Could you check a few things on this drawing? It's one solid part, dimensions in mm from its lowest x, y, z. A direction names the side the tool comes from. Round coordinates to 2 decimals unless told otherwise and drop trailing zeros. Write each loop counter-clockwise with the first axis right and the second up, starting at its lowest first coordinate (ties: lowest second). Pieces come first, ordered by that corner, then holes. Notation, with made-up numbers: (54.25, 20) -> (84.25, 20) arc R21 ccw to (84.25, 31) -> close; hole circle Ø7 at (70, -14.75). An arc over 180 degrees is marked (long way). Answer in a Markdown table with one row per item. Add a question column.
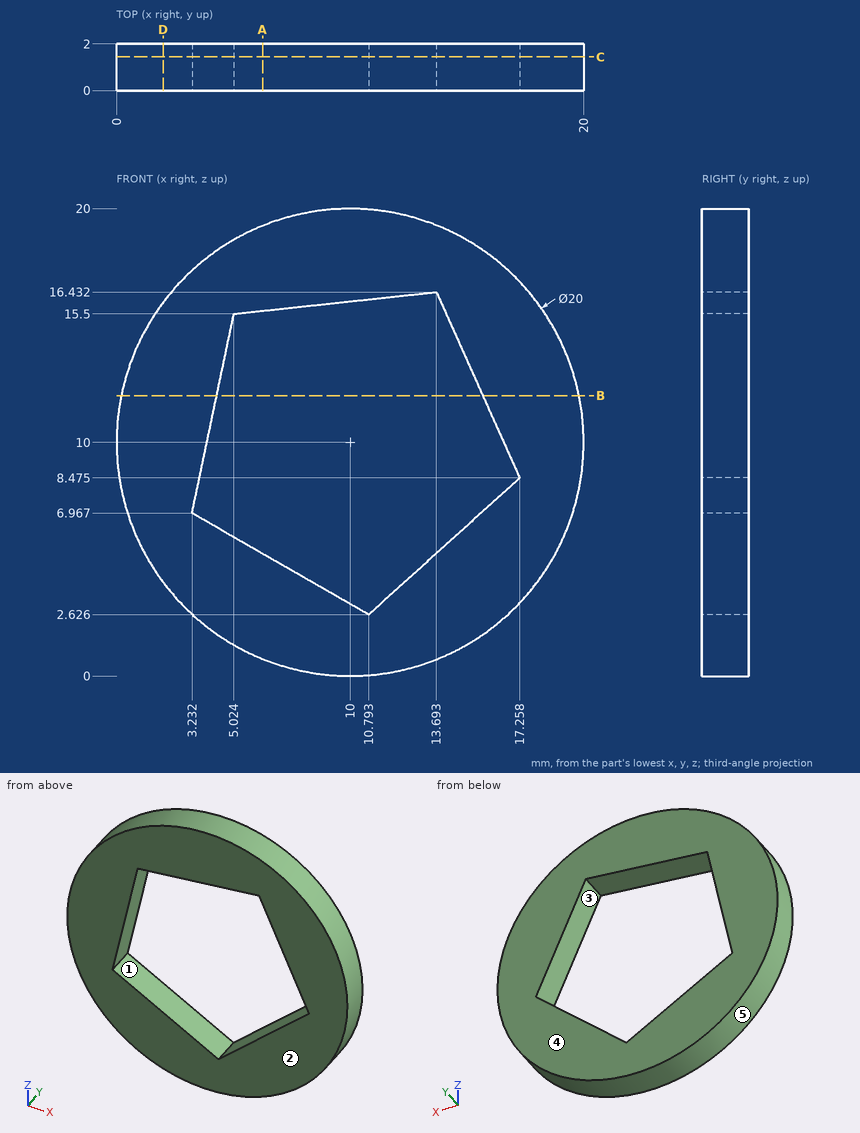
(1) I need wall thicknesses on L1, parallel to Z at x = 10.25, y = 0.35 (1 decimal); L2, parallel to Z at x = 13.5, y = 1.2 (1 decimal); L3, parallel to X at y = 1.7, z = 5 (1 decimal). Which ranges of each line are inside material? Lowest first, please.
(2) Suppose I cut it at B-B, the plane z = 12. Please give me the cut outline in (x, y), then the cut area to 3 significant figures.
(3) Suppose I cut it at C-C, the plane y = 1.45. Please give me the cut outline in (x, z) (1 decimal).
(4) If we mould it in two halves opening along X, with no side actions, what happens to the marked faces 3, 4 and 5? For each: pulls with the +X half, pulls with the -X half, needs draft (parallel to the pull), parting line crosses it, or undercut.
(5) On a 3-axis mill with a long thin cutter (end or side, diameter ignored), from which of +Z, -Z, +X, -X, +Y, -Y can I reach the whole of each face in a straight line? I mean the marked faces 1 and 2. Say none if no direction works.
(6) Suppose I cut it at D-D, the plane x = 2. Please give me the cut outline in (y, z).
(7) Suppose I cut it at A-A, the plane x = 6.25. Please give me the cut outline in (y, z) (1 decimal).
Response:
| question | item | result |
|---|---|---|
| 1 | L1 | 0 to 2.9, 16.1 to 20 |
| 1 | L2 | 0.6 to 5.1, 16.4 to 19.4 |
| 1 | L3 | 1.3 to 6.7, 13.4 to 18.7 |
| 2 | outline | (0.2, 0) -> (4.29, 0) -> (4.29, 2) -> (0.2, 2) -> close; (15.68, 0) -> (19.8, 0) -> (19.8, 2) -> (15.68, 2) -> close |
| 2 | area | 16.4 mm² |
| 3 | outline | circle Ø20 at (10, 10); hole (3.2, 7) -> (10.8, 2.6) -> (17.3, 8.5) -> (13.7, 16.4) -> (5, 15.5) -> close |
| 4 | face 3 | undercut |
| 4 | face 4 | needs draft |
| 4 | face 5 | parting line crosses it |
| 5 | face 1 | +Y, -Y |
| 5 | face 2 | +Z, -Z, +X, -X, -Y |
| 6 | outline | (0, 4) -> (2, 4) -> (2, 16) -> (0, 16) -> close |
| 7 | outline | (0, 0.7) -> (2, 0.7) -> (2, 5.2) -> (0, 5.2) -> close; (0, 15.6) -> (2, 15.6) -> (2, 19.3) -> (0, 19.3) -> close |
